Drawing for the job (mm, zero at the part's lowest x, y, z). A direction names the side the tool comes from. Coordinates: 2 decimals unless noted, no trailing zeros. Order: outer loops, then holes, each group sorted by start corner. A loop starts at its lowest first (then second) coordinate and runs counter-clockwise, first axis right, second up. Notation, with made-up numbers: (41.25, -1.5) -> (61.25, -1.5) arc R16 ccw to (61.25, 18.5) -> close; hole circle Ø10 at (56.25, -20). An arc over 180 degrees is marked (long way). Write each question's results on one line, items separated by ' | '.
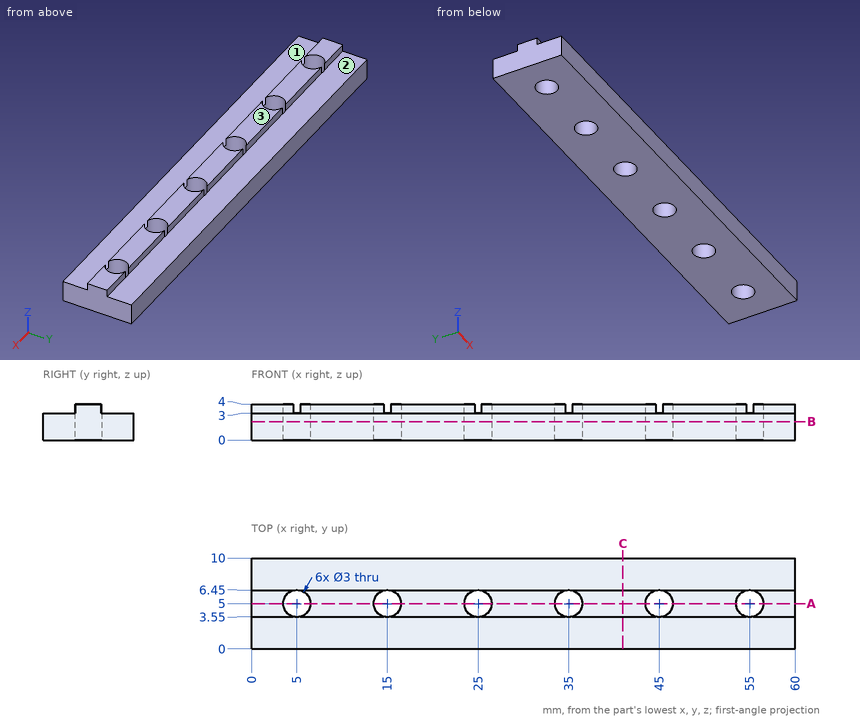
Item 1: Slice it at A-A, the plane y = 5. List the corners of the cut face in (x, z).
Answer:
outline: (0, 0) -> (3.5, 0) -> (3.5, 4) -> (0, 4) -> close; (6.5, 0) -> (13.5, 0) -> (13.5, 4) -> (6.5, 4) -> close; (16.5, 0) -> (23.5, 0) -> (23.5, 4) -> (16.5, 4) -> close; (26.5, 0) -> (33.5, 0) -> (33.5, 4) -> (26.5, 4) -> close; (36.5, 0) -> (43.5, 0) -> (43.5, 4) -> (36.5, 4) -> close; (46.5, 0) -> (53.5, 0) -> (53.5, 4) -> (46.5, 4) -> close; (56.5, 0) -> (60, 0) -> (60, 4) -> (56.5, 4) -> close
Item 2: Slice it at B-B, the plane z = 2.05. List the corners of the cut face in (x, y).
Answer:
outline: (0, 0) -> (60, 0) -> (60, 10) -> (0, 10) -> close; hole circle Ø3 at (5, 5); hole circle Ø3 at (15, 5); hole circle Ø3 at (25, 5); hole circle Ø3 at (35, 5); hole circle Ø3 at (45, 5); hole circle Ø3 at (55, 5)
Item 3: Pin check, flat tips, straight feed: pin 1 (2.5 mm diameter, centred on x = 35, y = 5, fed in from +Z); pin 2 (0.5 mm diameter, centred on x = 57.5, z = 3.5, fed in from +Y); pin 3 (4 mm diameter, centred on x = 24.5, y = 3.5, fed in from -Z); pin 4 (3 mm diameter, centred on x = 27, y = 2, fed in from +Z). Stop position of each tip, or through.
Answer:
pin 1: passes through | pin 2: stops at y = 6.45 | pin 3: stops at z = 0 | pin 4: stops at z = 3
Item 4: Tool access for the marked faces 1, 2 and 3: list every direction of +Z, -Z, +X, -X, +Y, -Y with a clear straight run to the whole face (end or side of a thin tool).
Answer:
face 1: +Z, +X, -X, -Y | face 2: +Z, +X, -X, +Y | face 3: +Z, +X, -X, +Y, -Y
Item 5: Drill centre lines: line 1 (Y direction, x = 5, z = 1); line 2 (Z direction, x = 57, y = 1.5); line 3 (Y direction, x = 11, z = 3.15). Where is each one in solid material? Low to high. Write a range as from..to.
Answer:
line 1: y = 0..3.5, 6.5..10 | line 2: z = 0..3 | line 3: y = 3.55..6.45
Item 6: Slice it at C-C, the plane x = 41. List the corners of the cut face in (y, z), and give its area (3 significant figures).
Answer:
outline: (0, 0) -> (10, 0) -> (10, 3) -> (6.45, 3) -> (6.45, 4) -> (3.55, 4) -> (3.55, 3) -> (0, 3) -> close | area: 32.9 mm^2
